Geometry check sheet. Reference: the model listing, model coordinates, mm. A direction names the side the tool comes from. Coordinates: 2 decimals unless noted, no trailing zeros. Order: outer loops, then holes, each group sorted by start corner. A loop starts at its lowest first (then second) coordinate and runs counter-clockwise, first axis right, second up. Notation, with made-up numbers: (40.25, -34) - (99.25, -34) arc R17 ccw to (99.25, -16) - close; hole circle Ø8 at (15, -32). An arc over 180 degrees is marked (long way). Put each result on its own line as item: value.
from build123d import *

# Parameters (mm, degrees)
SKETCH1_R           = 1.5
BOSS_EXTRUDE1_DEPTH = 3.175


with BuildPart() as part:
    # Sketch1 → Boss-Extrude1 (new body)
    with BuildSketch(Plane(origin=(0, 0, 0), x_dir=(1, 0, 0), z_dir=(0, 1, 0))):
        Polygon((35, 9.999999982), (20, 9.999999982), (20, -45), (35, -45), (35, -70), (-35, -70), (-35, 70), (35, 70), align=None)
        with Locations(Location((31, -62, 0), (0, 0, 270))):
            Circle(SKETCH1_R, mode=Mode.SUBTRACT)
        with Locations(Location((-31, -62, 0), (0, 0, 90))):
            Circle(SKETCH1_R, mode=Mode.SUBTRACT)
        with Locations(Location((-31, 62, 0), (0, 0, 270))):
            Circle(SKETCH1_R, mode=Mode.SUBTRACT)
        with Locations(Location((31, 62, 0), (0, 0, 90))):
            Circle(SKETCH1_R, mode=Mode.SUBTRACT)
    extrude(amount=BOSS_EXTRUDE1_DEPTH)


solid = part.part
Q1. Section check A-A on z = 62. Record the boundary of the cut face in (x, y) (3 decimals), then the cut area to 3 significant figures.
Answer block:
outline: (-35, 0) - (-32.5, 0) - (-32.5, 3.175) - (-35, 3.175) - close; (-29.5, 0) - (29.5, 0) - (29.5, 3.175) - (-29.5, 3.175) - close; (32.5, 0) - (35, 0) - (35, 3.175) - (32.5, 3.175) - close
area: 203 mm^2
Q2. Thickness scan on L1, parallel to X at y = 1.65, z = 62; L2, parallel to Z at x = 23, y = 1.9; L3, parallel to Z at x = 30, y = 3. Record the ranges inside material, lowest first. Write a range as [from, to].
Answer block:
L1: x = [-35, -32.5], [-29.5, 29.5], [32.5, 35]
L2: z = [-70, -10], [45, 70]
L3: z = [-70, -63.12], [-60.88, -10], [45, 60.88], [63.12, 70]
Q3. Section check C-C on y = 1.8. Record the boundary of the cut face in (x, z), then the cut area to 3 significant figures.
Answer block:
outline: (-35, -70) - (35, -70) - (35, -10) - (20, -10) - (20, 45) - (35, 45) - (35, 70) - (-35, 70) - close; hole circle Ø3 at (-31, -62); hole circle Ø3 at (-31, 62); hole circle Ø3 at (31, -62); hole circle Ø3 at (31, 62)
area: 8,950 mm^2
Q4. Depth check by flat-ended pin: pin 1 Ø2.5 at (x, z) = (-31, 62) entering from -Y; pin 2 Ø3.5 at (x, z) = (31, 62) entering from +Y (3 decimals); pin 3 Ø1 at (y, z) = (2, 20.5) entering from +X. Enter the tip coordinate at first touch or a pass-through.
Answer block:
pin 1: passes through
pin 2: stops at y = 3.175
pin 3: stops at x = 20
Q5. Section check D-D on x = 31. Record the boundary of the cut face in (y, z) (3 decimals).
Answer block:
outline: (0, -70) - (3.175, -70) - (3.175, -63.5) - (0, -63.5) - close; (0, -60.5) - (3.175, -60.5) - (3.175, -10) - (0, -10) - close; (0, 45) - (3.175, 45) - (3.175, 60.5) - (0, 60.5) - close; (0, 63.5) - (3.175, 63.5) - (3.175, 70) - (0, 70) - close
Q6. Access from +Z, -Z, +X, -X, +Y, -Y to the whole of each face (thin tool, end or side, straight path). Record for faces 5 (the flat face through (20, 2, 17)), 6 (the flat face through (0, 0, -1)).
Answer block:
face 5: +X, +Y, -Y
face 6: +Z, -Z, +X, -X, -Y
Q7. Section check B-B on x = -31. Record the boundary of the cut face in (y, z) (3 decimals).
Answer block:
outline: (0, -70) - (3.175, -70) - (3.175, -63.5) - (0, -63.5) - close; (0, -60.5) - (3.175, -60.5) - (3.175, 60.5) - (0, 60.5) - close; (0, 63.5) - (3.175, 63.5) - (3.175, 70) - (0, 70) - close
Q8. Draft check along Z on faces 1 (the flat face through (0, 2, -70)), 2 (the flat face through (35, 2, -40)), 3 (the cylindrical face through (-30.55, 1.57, -60.57)), 4 (the flat face through (27, 2, 45)). Enter one of: pulls with the +Z half, pulls with the -Z half, needs draft (parallel to the pull), parting line crosses it, or undercut.
Answer block:
face 1: pulls with the -Z half
face 2: needs draft
face 3: undercut
face 4: undercut
